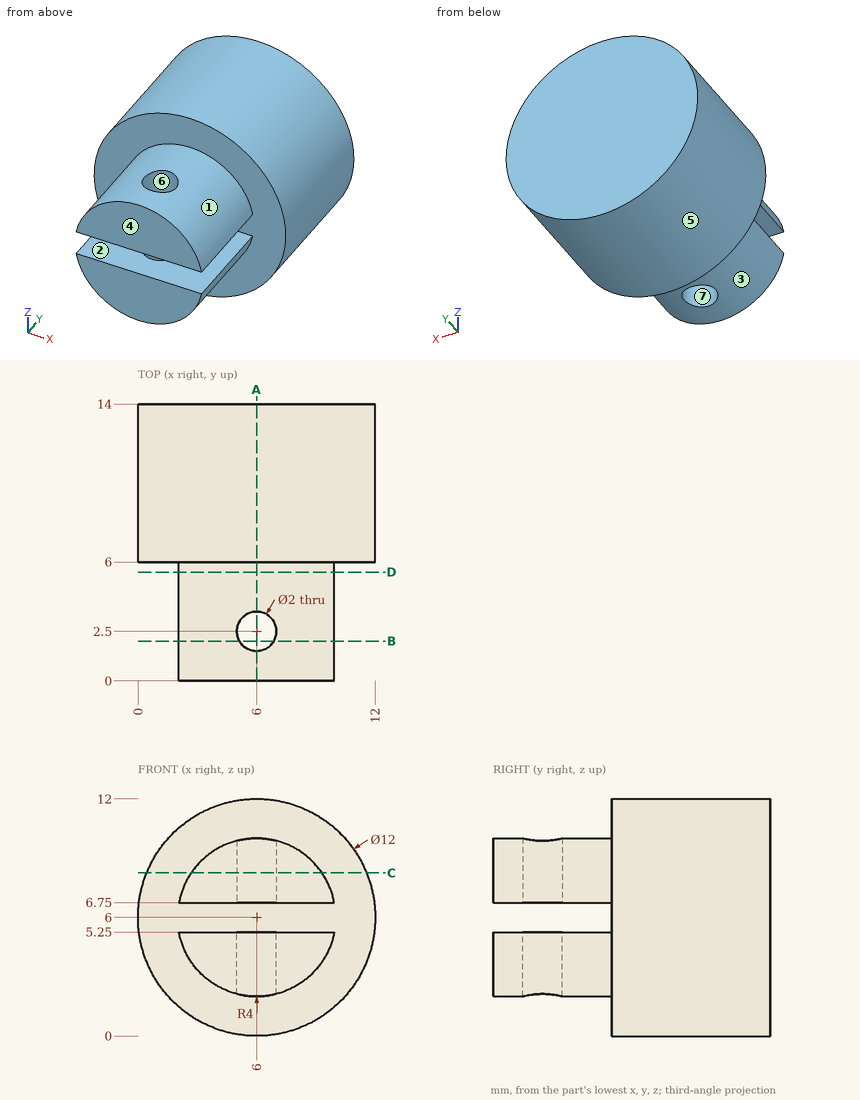
Study the drawing (mm; zero at the part's minimum x, y, z) and answer. A direction names the side the tool comes from. Round coordinates to 2 decimals unless told otherwise and drop trailing zeros. Loops run counter-clockwise (first coordinate to the right, second up) from the corner with the lowest first, then second, coordinate; pieces in that order, holes last.
Q1. For a pull along X with two mould halves and no side action, classify the marked faces 4, 5, 6 and 7 as released by +X, released by -X, zero draft, split by the parting line, or undercut.
Q2. Given pin 1 Ø6.5 at (x, y) = (7.5, 2) entering from -Z; pin 2 Ø1.5 at (y, z) = (12, 7) entering from +X; pin 3 Ø1 at (x, z) = (1.5, 9) entering from -Y, each flat-ended and moving along its own axis, determine where each tip first touches the part or whether it passes through.
Q3. Which of the six approach directions +Z, -Z, +X, -X, +Y, -Y give full straight-line access (tool end or side, diameter ignored) to the marked faces 1, 2 and 3?
Q4. Section C-C, the plane z = 8.25 is taken. Determine the outline of the cut face in (x, y), then the cut area to 3 significant figures.
Q5. Find the intervals of material crossed by line 1 (Y direction, x = 6, z = 3.6); line 2 (Z direction, x = 9.5, y = 5.5); line 3 (Y direction, x = 10.75, z = 7.5), in increasing order.
Q6. Section B-B, the plane y = 2 is taken. Determine the outline of the cut face in (x, z), then the cut area to 3 significant figures.
Q7. Section D-D, the plane y = 5.5 is taken. Determine the outline of the cut face in (x, z).
Q8. Section A-A, the plane x = 6 is taken. Determine the outline of the cut face in (y, z), then the cut area to 3 significant figures.
Completed:
1. face 4: zero draft
1. face 5: split by the parting line
1. face 6: undercut
1. face 7: undercut
2. pin 1: stops at z = 2
2. pin 2: stops at x = 11.99
2. pin 3: stops at y = 6
3. face 1: +Z, -Y
3. face 2: +X, -X, -Y
3. face 3: -Z, -Y
4. outline: (0.44, 6) - (2.69, 6) - (2.69, 0) - (9.31, 0) - (9.31, 6) - (11.56, 6) - (11.56, 14) - (0.44, 14) - close; hole circle Ø2 at (6, 2.5)
4. area: 126 mm2
5. line 1: y = 0 to 1.5, 3.5 to 14
5. line 2: z = 4.06 to 5.25, 6.75 to 7.94
5. line 3: y = 6 to 14
6. outline: (2.07, 5.25) arc R4 ccw to (5.13, 2.09) - (5.13, 5.25) - close; (2.07, 6.75) - (5.13, 6.75) - (5.13, 9.91) arc R4 ccw to start; (6.87, 2.09) arc R4 ccw to (9.93, 5.25) - (6.87, 5.25) - close; (6.87, 6.75) - (9.93, 6.75) arc R4 ccw to (6.87, 9.91) - close
6. area: 27.2 mm2
7. outline: (2.07, 5.25) arc R4 ccw to (9.93, 5.25) - close; (2.07, 6.75) - (9.93, 6.75) arc R4 ccw to start
8. outline: (0, 2) - (1.5, 2) - (1.5, 5.25) - (0, 5.25) - close; (0, 6.75) - (1.5, 6.75) - (1.5, 10) - (0, 10) - close; (3.5, 2) - (6, 2) - (6, 0) - (14, 0) - (14, 12) - (6, 12) - (6, 10) - (3.5, 10) - (3.5, 6.75) - (6, 6.75) - (6, 5.25) - (3.5, 5.25) - close
8. area: 122 mm2
